```python
from build123d import *

# Parameters (mm, degrees)
SKETCH1_W               = 75
SKETCH1_H               = 75
SKETCH1_R               = 3
SKETCH1_R_2             = 6
BOSS_EXTRUDE1_DEPTH     = 10
SKETCH2_W               = 10
SKETCH2_H               = 54.30825561
BOSS_EXTRUDE2_DEPTH     = 60
CUT_EXTRUDE1_DEPTH      = 110.230261375
CUT_EXTRUDE1_DEPTH_BACK = 110.230261375
SKETCH3_R               = 10
CUT_EXTRUDE2_DEPTH      = 81.07808689
CUT_EXTRUDE2_DEPTH_BACK = 81.07808689
SKETCH5_W               = 55
SKETCH5_H               = 20
CUT_EXTRUDE3_DEPTH      = 5


with BuildPart() as part:
    # Sketch1 → Boss-Extrude1 (new body)
    with BuildSketch(Plane(origin=(0, 0, 0), x_dir=(1, 0, 0), z_dir=(0, 1, 0))):
        Rectangle(SKETCH1_W, SKETCH1_H)
        with Locations(Location((-32.66, 32.72, 0), (0, 0, 270))):
            Circle(SKETCH1_R, mode=Mode.SUBTRACT)
        with Locations(Location((32.66, 32.72, 0), (0, 0, 90))):
            Circle(SKETCH1_R, mode=Mode.SUBTRACT)
        with Locations(Location((32.66, -32.72, 0), (0, 0, 270))):
            Circle(SKETCH1_R, mode=Mode.SUBTRACT)
        with Locations(Location((-32.66, -32.72, 0), (0, 0, 90))):
            Circle(SKETCH1_R, mode=Mode.SUBTRACT)
        with Locations(Location((0, 0, 0), (0, 0, 270))):
            Circle(SKETCH1_R_2, mode=Mode.SUBTRACT)
    extrude(amount=BOSS_EXTRUDE1_DEPTH)

    # Sketch2 → Boss-Extrude2 (add)
    with BuildSketch(Plane(origin=(0, 10, 0), x_dir=(1, 0, 0), z_dir=(0, 1, 0))):
        with Locations((-32.5, 0)):
            Rectangle(SKETCH2_W, SKETCH2_H)
        with Locations((32.5, 0)):
            Rectangle(SKETCH2_W, SKETCH2_H)
    extrude(amount=BOSS_EXTRUDE2_DEPTH)

    # Sketch3 → Cut-Extrude1 (cut, two sides: drawn at the far end of the back side and taken through both)
    with BuildSketch(Plane.ZY.offset(37.5).offset(-CUT_EXTRUDE1_DEPTH_BACK)):
        with Locations((0, 40)):
            Circle(SKETCH3_R)
    extrude(amount=CUT_EXTRUDE1_DEPTH + CUT_EXTRUDE1_DEPTH_BACK, mode=Mode.SUBTRACT)

    # Sketch4 → Cut-Extrude2 (cut, two sides: drawn at the far end of the back side and taken through both)
    with BuildSketch(Plane(origin=(0, 10, 0), x_dir=(1, 0, 0), z_dir=(0, 1, 0)).offset(-CUT_EXTRUDE2_DEPTH_BACK)):
        Polygon((-27.5, 10), (27.5, 10), (27.5, 27.154127805), (27.5, 37.5), (-27.5, 37.5), (-27.5, 27.154127805), align=None)
        Polygon((27.5, -27.154127805), (27.5, -10), (-27.5, -10), (-27.5, -27.154127805), (-27.5, -37.5), (27.5, -37.5), align=None)
    extrude(amount=CUT_EXTRUDE2_DEPTH + CUT_EXTRUDE2_DEPTH_BACK, mode=Mode.SUBTRACT)

    # Sketch5 → Cut-Extrude3 (cut)
    with BuildSketch(Plane(origin=(0, 10, 0), x_dir=(1, 0, 0), z_dir=(0, 1, 0))):
        Rectangle(SKETCH5_W, SKETCH5_H)
    extrude(amount=-CUT_EXTRUDE3_DEPTH, mode=Mode.SUBTRACT)


solid = part.part
```
Geometry: final body of the model. Coordinates: model frame, mm. A direction names the side the tool comes from. Round coordinates to 2 decimals unless told otherwise and drop trailing zeros. Order: outer loops, then holes, each group sorted by start corner. A loop starts at its lowest first (then second) coordinate and runs counter-clockwise, first axis right, second up. Notation, with made-up numbers: M 72.25,48 L 131.25,48 A22 cw 131.25,62 Z; hole C 36.5,10 d5. An arc over 180 degrees is marked long. Use one line per item in the form item = value. Start each with the question number.
Q1. Cut plane C-C (y = 40). Return loops of the section in (x, z).
Q2. Cut plane A-A (x = -32.66). Return loops of the section in (y, z).
Q3. Cut plane D-D (z = 0). Return loops of the section in (x, y).
Q4. Access query for faces 1 (the face through (-6.5, 5, -0.1)), 2 (the face through (0, 2, -10)), 3 (the face through (32, 40, 27.154)). Directions: +Z, -Z, +X, -X, +Y, -Y. A direction counts if a zero-diameter tool reaches every point of the face in a straight line with its end or side. Return the directions, or none.
Q5. Material intervals for line 1 (X direction, y = 4.75, z = 32.72); line 2 (Y direction, x = -32.5, z = 0); line 3 (X direction, y = 25.5, z = 11), sorted ascending. Write a range as [from, to].
Q6. Cut plane B-B (z = 20). Return loops of the section in (x, y).
Q7. Mould query, pull axis Y, two halves, no side actions, for faces 4 (the face through (-32.43, 30.24, -2.17)), 5 (the face through (-33, 5, -37.5)), 6 (the face through (-1, 0, -9)). Classes: +Y half, -Y half, draft (parallel to the pull), parting line (faces both ways), or undercut.
Q8. Pin query (flat end, axial travel): pin 1 Ø11 at (x, y) = (33.5, 38) entering from -Z; pin 2 Ø3.5 at (x, z) = (32.66, -32.72) entering from +Y; pin 3 Ø3 at (x, z) = (-34, 30) entering from +Y; pin 4 Ø5 at (x, y) = (-33, 30.5) entering from +Z. Return the tip coordinate at first contact, or that it passes through.
Geometry results:
q1.outline = M -37.5,-27.15 L -27.5,-27.15 L -27.5,-10 L -37.5,-10 Z; M -37.5,10 L -27.5,10 L -27.5,27.15 L -37.5,27.15 Z; M 27.5,-27.15 L 37.5,-27.15 L 37.5,-10 L 27.5,-10 Z; M 27.5,10 L 37.5,10 L 37.5,27.15 L 27.5,27.15 Z
q2.outline = M 0,-37.5 L 10,-37.5 L 10,-35.72 L 0,-35.72 Z; M 0,-29.72 L 10,-29.72 L 10,-27.15 L 70,-27.15 L 70,27.15 L 10,27.15 L 10,29.72 L 0,29.72 Z; M 0,35.72 L 10,35.72 L 10,37.5 L 0,37.5 Z; hole C 40,0 d20
q3.outline = M -37.5,0 L -6,0 L -6,5 L -27.5,5 L -27.5,30 L -37.5,30 Z; M -37.5,50 L -27.5,50 L -27.5,70 L -37.5,70 Z; M 6,0 L 37.5,0 L 37.5,30 L 27.5,30 L 27.5,5 L 6,5 Z; M 27.5,50 L 37.5,50 L 37.5,70 L 27.5,70 Z
q4.face_1 = +Z, -Z, +Y
q4.face_2 = -Z, +Y, -Y
q4.face_3 = +Z, +X, -X, +Y
q5.line_1 = [-37.5, -35.66], [-29.66, -27.5], [27.5, 29.66], [35.66, 37.5]
q5.line_2 = [0, 30], [50, 70]
q5.line_3 = [-37.5, -27.5], [27.5, 37.5]
q6.outline = M -37.5,0 L -27.5,0 L -27.5,70 L -37.5,70 Z; M 27.5,0 L 37.5,0 L 37.5,70 L 27.5,70 Z
q7.face_4 = undercut
q7.face_5 = draft
q7.face_6 = -Y half
q8.pin_1 = -27.15
q8.pin_2 = through
q8.pin_3 = 10
q8.pin_4 = 27.15
